Source: CAD feature listing. Evaluate the final solid. Frame: model axes, mm. Face numbers are marked on the shaded views. Round coordinates to 2 decimals unless told otherwise and drop trailing zeros. Write each loop counter-clockwise with the first axis right and the second up, starting at its lowest first coordinate (ties: lowest second). Pieces come first, ordered by that corner, then holes. Notation, with made-up numbers: (-23, 9.25) - (-18, 9.25) arc R25 ccw to (-18, 31.25) - close; hole circle Ø9 at (54.25, 2.5). An arc over 180 degrees is marked (long way). Write item = value, one per line. Start each with the question number.
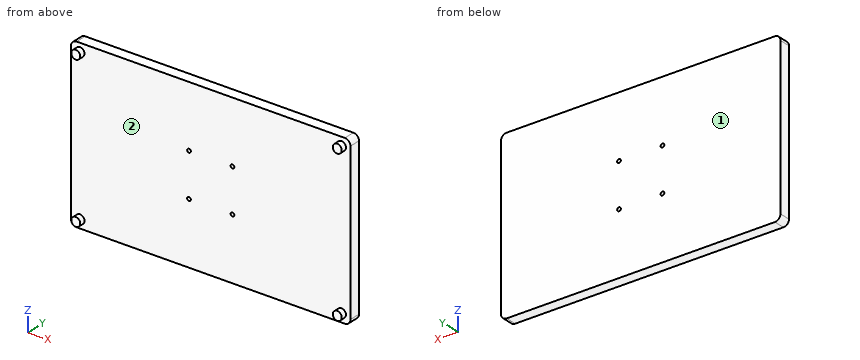
```python
from build123d import *

# Parameters (mm, degrees)
BOSS_EXTRUDE1_DEPTH     = 20
CUT_EXTRUDE2_DEPTH      = 20
CUT_EXTRUDE2_DEPTH_BACK = 293.232783924
SKETCH2_R               = 3.3
SKETCH3_R               = 8
BOSS_EXTRUDE2_DEPTH     = 10


with BuildPart() as part:
    # Sketch1 → Boss-Extrude1 (new body)
    with BuildSketch(Plane(origin=(0, 0, 0), x_dir=(1, 0, 0), z_dir=(0, 1, 0))):
        with BuildLine():
            Line((240, -150), (-240, -150))
            ThreePointArc((-240, -150), (-247.071067812, -147.071067812), (-250, -140))
            Line((-250, -140), (-250, 140))
            ThreePointArc((-250, 140), (-247.071067812, 147.071067812), (-240, 150))
            Line((-240, 150), (240, 150))
            ThreePointArc((240, 150), (247.071067812, 147.071067812), (250, 140))
            Line((250, 140), (250, -140))
            ThreePointArc((250, -140), (247.071067812, -147.071067812), (240, -150))
        make_face()
    extrude(amount=BOSS_EXTRUDE1_DEPTH)

    # Sketch2 → Cut-Extrude2 (cut, two sides: drawn at the far end of the back side and taken through both)
    with BuildSketch(Plane(origin=(0, 0, 0), x_dir=(1, 0, 0), z_dir=(0, 1, 0)).offset(-CUT_EXTRUDE2_DEPTH_BACK)):
        with Locations(Location((-38.87, -38.87, 0), (0, 0, 270))):
            Circle(SKETCH2_R)
        with Locations(Location((38.87, -38.87, 0), (0, 0, 270))):
            Circle(SKETCH2_R)
        with Locations(Location((38.87, 38.87, 0), (0, 0, 270))):
            Circle(SKETCH2_R)
        with Locations(Location((-38.87, 38.87, 0), (0, 0, 270))):
            Circle(SKETCH2_R)
    extrude(amount=CUT_EXTRUDE2_DEPTH + CUT_EXTRUDE2_DEPTH_BACK, mode=Mode.SUBTRACT)

    # Sketch3 → Boss-Extrude2 (add)
    with BuildSketch(Plane(origin=(0, 0, 0), x_dir=(1, 0, 0), z_dir=(0, 1, 0))):
        with Locations(Location((-234, 135, 0), (0, 0, 270))):
            Circle(SKETCH3_R)
        with Locations(Location((234, 135, 0), (0, 0, 270))):
            Circle(SKETCH3_R)
        with Locations(Location((234, -135, 0), (0, 0, 270))):
            Circle(SKETCH3_R)
        with Locations(Location((-234, -135, 0), (0, 0, 270))):
            Circle(SKETCH3_R)
    extrude(amount=-BOSS_EXTRUDE2_DEPTH)


solid = part.part
```
(1) Section A-A (x = -234). Return the cut outline in (y, z).
(2) Contact query for flat-ended pins moving along their axis: P1, Ø3, axis at x = -91, z = 105.5, coming from the -Y side; P2, Ø10.5, axis at x = 38.87, z = -38.87, coming from the +Y side. Output: stop coordinate, or through.
(3) Section B-B (z = -135). Return the cut outline in (x, y).
(4) Section C-C (z = 69). Return the cut outline in (x, y), plus the area to 3 significant figures.
(5) Pull-direction query (X, two-part tool) for the marked faces 1 and 2; classes: +X half, -X half, draft (parallel to the pull), parting line (faces both ways), or undercut.
(6) Ray query, L1, parallel to X at y = 14.75, z = -38.87; L2, parallel to Z at x = -38.87, y = 10.5; L3, parallel to Y at x = -72, z = 44.5. Return the intervals inside material, ascending. Write a range as from..to.
Solution:
q1.outline = (-10, -143) - (0, -143) - (0, -150) - (20, -150) - (20, 150) - (0, 150) - (0, 143) - (-10, 143) - (-10, 127) - (0, 127) - (0, -127) - (-10, -127) - close
q2.P1 = 0
q2.P2 = 20
q3.outline = (-250, 0) - (-242, 0) - (-242, -10) - (-226, -10) - (-226, 0) - (226, 0) - (226, -10) - (242, -10) - (242, 0) - (250, 0) - (250, 20) - (-250, 20) - close
q4.outline = (-250, 0) - (250, 0) - (250, 20) - (-250, 20) - close
q4.area = 10,000 mm^2
q5.face_1 = draft
q5.face_2 = undercut
q6.L1 = -250..-42.17, -35.57..35.57, 42.17..250
q6.L2 = -150..-42.17, -35.57..35.57, 42.17..150
q6.L3 = 0..20
